Part print with two shaded views. Sizes in mm from the minimum x, y, z corner. A direction names the side the tool comes from. Round coordinates to 2 decimals unless told otherwise and drop trailing zeros. Loops run counter-clockwise (first coordinate to the right, second up) from the corner with the lowest first, then second, coordinate; pieces in that order, holes last. Notation, with made-up numbers: (23, 86.25) -> (77, 86.25) arc R31 ccw to (77, 118.25) -> close; hole circle Ø6 at (23, -13). An arc over 180 degrees is marked (long way). Use a Markdown table: item, result. Add a question column.
Item 1: Cut at A-A, the plane z = 122. List the corners of the cut face in (x, y).
Item 2: Cut at D-D, the plane y = 56. List the corners of the cut face in (x, z).
Item 3: Probe line 1 (X direction, y = 239, z = 322.5); line 2 (Z direction, x = 263.5, y = 309); line 3 (Y direction, x = 486, z = 178.5). List the from-to ranges inside material, lowest first. Write a range as [from, to].
Item 4: Two-plate mould, pull along X, no slides. Class the marked faces 3, 4 and 5: pulls with the +X half, pulls with the -X half, needs draft (parallel to the pull), parting line crosses it, or undercut.
Item 5: Cut at B-B, the plane y = 325. List the corners of the cut face in (x, z), plus the area to 3 significant figures.
Item 6: Cut at C-C, the plane x = 280.5. List the corners of the cut face in (y, z).
Item 7: Which spindle directions (+Z, -Z, +X, -X, +Y, -Y) get a long thin tool onto all of the face, cutting with end or side? Do the marked faces 1 and 2. Say none if no direction does.
Item 8: Flat gauge pins, fed straight in: pin 1 (3 mm diameter, centred on x = 2, z = 219, fed in from -Y); pin 2 (1.9 mm diameter, centred on y = 33, z = 4.5, fed in from +X); pin 3 (5 mm diameter, centred on x = 161, z = 339, fed in from -Y); pin 4 (5 mm diameter, centred on y = 73.5, z = 234.5, fed in from -X). Where does each tip first touch, or does it go through?
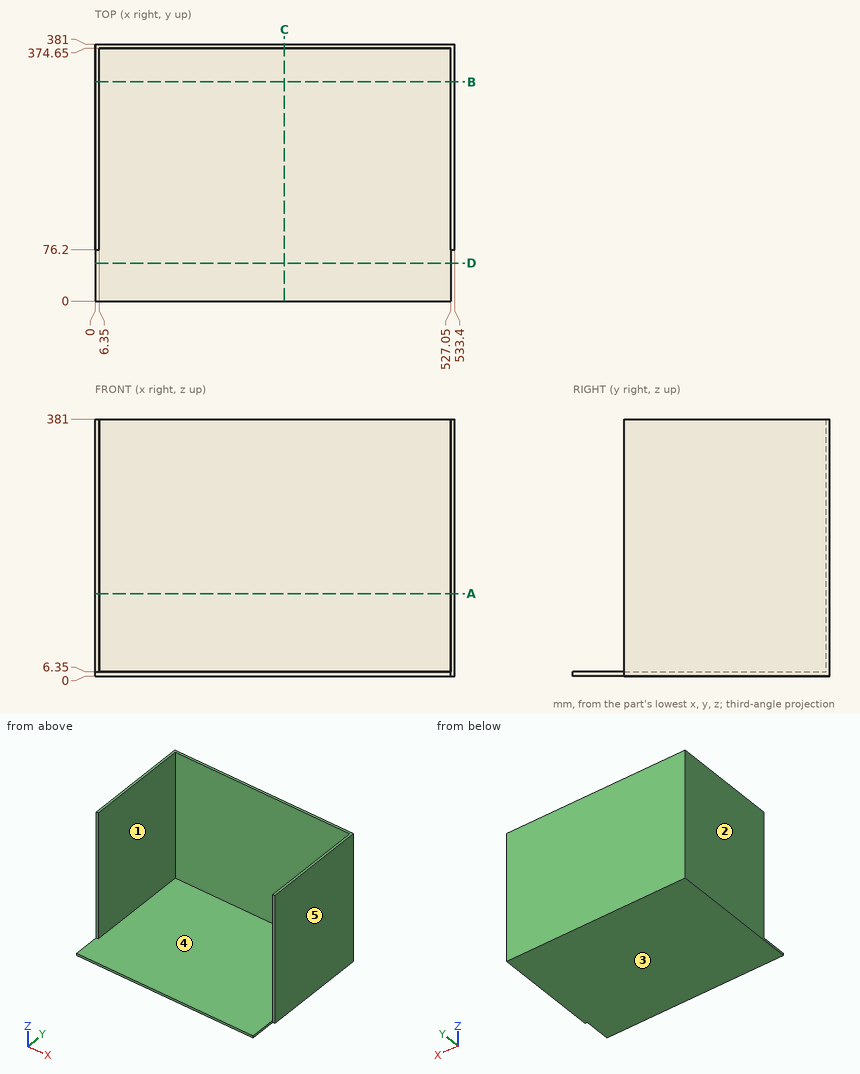
A:
| question | item | result |
|---|---|---|
| 1 | outline | (0, 76.2) -> (6.35, 76.2) -> (6.35, 374.65) -> (527.05, 374.65) -> (527.05, 76.2) -> (533.4, 76.2) -> (533.4, 381) -> (0, 381) -> close |
| 2 | outline | (0, 0) -> (527.05, 0) -> (527.05, 6.35) -> (0, 6.35) -> close |
| 3 | line 1 | x = [0, 6.35], [527.05, 533.4] |
| 3 | line 2 | z = [0, 6.35] |
| 3 | line 3 | y = [374.65, 381] |
| 4 | face 3 | needs draft |
| 4 | face 4 | undercut |
| 4 | face 5 | pulls with the +X half |
| 5 | outline | (0, 0) -> (533.4, 0) -> (533.4, 381) -> (527.05, 381) -> (527.05, 6.35) -> (6.35, 6.35) -> (6.35, 381) -> (0, 381) -> close |
| 5 | area | 8,150 mm^2 |
| 6 | outline | (0, 0) -> (381, 0) -> (381, 381) -> (374.65, 381) -> (374.65, 6.35) -> (0, 6.35) -> close |
| 7 | face 1 | +Z, -Y |
| 7 | face 2 | +Z, -Z, -X, +Y, -Y |
| 8 | pin 1 | stops at y = 76.2 |
| 8 | pin 2 | stops at x = 527.05 |
| 8 | pin 3 | stops at y = 374.65 |
| 8 | pin 4 | passes through |
